For this review, take the finished solid that the model builds, in its own axes (mm). Coordinates: 2 decimals unless noted, no trailing zeros. Order: outer loops, then holes, each group sorted by start corner. A loop starts at its lowest first (then second) coordinate and runs counter-clockwise, first axis right, second up.
Autodesk Inventor part; units mm, degrees
ref_plane "YZ Plane" through (0, 0, 0) normal (1, 0, 0) x (0, 1, 0)
ref_plane "XZ Plane" through (0, 0, 0) normal (0, 1, 0) x (-1, 0, 0)
ref_plane "XY Plane" through (0, 0, 0) normal (0, 0, 1) x (1, 0, 0)
sketch "Sketch1" plane through (0, 0, 0) normal (0, 0, 1) x (1, 0, 0)
  circle A0 centre (-86.3708, -61.0441) radius 4.8895
  circle A1 centre (-86.3708, -61.0441) radius 4.8895
  line L0 (-81.8807, -65.5342) -> (40.0712, 56.4176)
  line L1 (31.091, 65.3979) -> (-90.8609, -56.554)
  arc A2 (-90.8609, -56.554) -> (-81.8807, -65.5342) centre (-86.3708, -61.0441) ccw
  arc A3 (40.0712, 56.4176) -> (31.091, 65.3979) centre (35.5811, 60.9078) ccw
  circle A4 centre (-25.3948, -0.0682) radius 4.8895
  circle A5 centre (35.5811, 60.9078) radius 4.8895
  line L2 (-21.9374, 3.3892) -> (32.1237, 57.4504)
  line L3 (39.0385, 64.3652) -> (40.0712, 65.3979)
  line L4 (-82.9134, -57.5867) -> (-28.8522, -3.5256) construction
  line L5 (-21.9374, 3.3892) -> (32.1237, 57.4504) construction
  line L6 (-28.8522, -3.5256) -> (-82.9134, -57.5867)
  line L7 (-89.8282, -64.5015) -> (-90.8609, -65.5342)
  line L8 (-34.6701, -9.3434) -> (-77.0956, -51.7689) construction
  line L9 (-37.2209, -6.7925) -> (-79.6465, -49.218)
  line L10 (-74.5447, -54.3198) -> (-32.1192, -11.8943)
  arc A6 (-32.1192, -11.8943) -> (-37.2209, -6.7925) centre (-34.6701, -9.3434) ccw
  arc A7 (-79.6465, -49.218) -> (-74.5447, -54.3198) centre (-77.0956, -51.7689) ccw
  line L11 (-25.3948, -0.0682) -> (-29.885, 4.422)
  line L12 (-18.6705, 11.7579) -> (23.755, 54.1835)
  line L13 (28.8568, 49.0817) -> (-13.5688, 6.6562)
  arc A8 (-18.6705, 11.7579) -> (-13.5688, 6.6562) centre (-16.1196, 9.207) ccw
  arc A9 (28.8568, 49.0817) -> (23.755, 54.1835) centre (26.3059, 51.6326) ccw
  line L14 (40.9692, 55.5196) -> (-80.9826, -66.4323)
  arc A10 (-91.7589, -55.6559) -> (-80.9826, -66.4323) centre (-86.3708, -61.0441) ccw
  line L15 (-91.7589, -55.6559) -> (30.1929, 66.2959)
  arc A11 (40.9692, 55.5196) -> (30.1929, 66.2959) centre (35.5811, 60.9078) ccw
  point P0 (0, 0)
  point P1 (-55.8828, -30.5561)
  dimension "d0" = 172.466
  dimension "d2" = 12.7
  dimension "d5" = 9.779
  dimension "d6" = 9.779
  dimension "d7" = 9.779
  dimension "d10" = 1.27
extrude "Extrusion1" add sketch "Sketch1" along normal blind 7.62 contours A0 L6 A7 L10 A6 A4 L2 A8 L13 A9 A5 L3 A3 L0 A2 L7 | A0 L7 A2 L1 L11 A4 L6 A6 L9 A7 | L1 A3 L3 A5 L2 A9 L12 A8 A4 L11
extrude "Extrusion2" add sketch "Sketch1" along normal up to surface (7.62 mm away)
properties part number "Reg Arm"
1. Take a section at A-A, the plane z = 3.25. Give the boundary of the cut face in (x, y) (1 decimal), plus the area to 3 significant figures.
Answer below:
outline: (-91.8, -55.7) arc R7.6 ccw to (-81, -66.4) - (41, 55.5) arc R7.6 ccw to (30.2, 66.3) - close; hole circle Ø9.8 at (-86.4, -61); hole (-79.6, -49.2) arc R3.6 ccw to (-74.5, -54.3) - (-32.1, -11.9) arc R3.6 ccw to (-37.2, -6.8) - close; hole circle Ø9.8 at (-25.4, -0.1); hole (-18.7, 11.8) arc R3.6 ccw to (-13.6, 6.7) - (28.9, 49.1) arc R3.6 ccw to (23.8, 54.2) - close; hole circle Ø9.8 at (35.6, 60.9)
area: 1,640 mm2
2. The part is to be moulded in two halves that separate along X. For faces 1 (the face through (-19.15, -4.6, 3.76)), 2 (the face through (2.245, 32.674, 3.757)), 3 (the face through (-31.637, 4.466, 3.757)), 4 (the face through (-53.629, -33.404, 3.757)), say which applies: +X half, -X half, draft (parallel to the pull), parting line (faces both ways), or undercut.
Answer below:
face 1: +X half
face 2: undercut
face 3: -X half
face 4: undercut
3. To check wall thickness, follow L1, parallel to Y at x = -54.5, z = 7; L2, parallel to X at y = -8, z = 2.25; L3, parallel to Y at x = -69.5, z = 5. State the ranges of each line that lie inside material, in increasing order.
Answer below:
L1: y = -39.95 to -34.28, -24.07 to -18.4
L2: x = -44.1 to -38.43, -31.32 to -22.55
L3: y = -54.95 to -49.28, -39.07 to -33.4
4. Take a section at C-C, the plane y = 26. Give the boundary of the cut face in (x, z).
Answer below:
outline: (-10.1, 0) - (-4.43, 0) - (-4.43, 7.62) - (-10.1, 7.62) - close; (5.78, 0) - (11.45, 0) - (11.45, 7.62) - (5.78, 7.62) - close
5. Take a section at B-B, the plane x = 2. Give the boundary of the cut face in (y, z), plus the area to 3 significant figures.
Answer below:
outline: (16.55, 0) - (22.22, 0) - (22.22, 7.62) - (16.55, 7.62) - close; (32.43, 0) - (38.1, 0) - (38.1, 7.62) - (32.43, 7.62) - close
area: 86.5 mm2
6. Clearance check with flat-ended pins moving along their axes: pin 1 Ø1.5 at (x, z) = (-12, 1.5) entering from +Y; pin 2 Ø4 at (y, z) = (-35.5, 5.5) entering from +X. State where each tip first meets the part, or that it passes through.
Answer below:
pin 1: stops at y = 24.85
pin 2: stops at x = -48.05
